Source: CAD feature listing. Evaluate the final solid. Frame: model axes, mm. Face numbers are marked on the shaded views. A direction names the side the tool comes from. Round coordinates to 2 decimals unless told otherwise and drop trailing zeros. Write each loop counter-clockwise with the first axis right and the second up, starting at its lowest first coordinate (ties: lowest second). Pieces come first, ordered by that corner, then holes. Notation, with made-up numbers: M 71.5,29 L 101.5,29 A19 ccw 101.5,45 Z; hole C -8,12.5 d10. An arc over 180 degrees is marked long. Use a Markdown table: item, result.
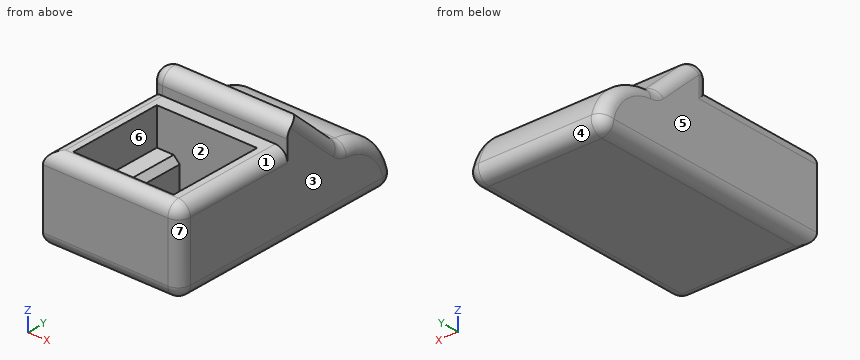
```python
from build123d import *

# Parameters (mm, degrees)
F0_W     = 57.6730370522
F0_H     = 103.7285923958
F1_DEPTH = 50.1204133034
F2_W     = 51.8642961979
F2_H     = 15.2675881982
F3_DEPTH = 280.9666395187
F4_W     = 42.251765728
F4_H     = 40.2974346653
F5_DEPTH = 28.219755739
F6_W     = 9.6290325746
F6_H     = 40.2974346653
F7_DEPTH = 12.7694699913
F8_W     = 9.6542518586
F8_H     = 40.2974346653
F9_DEPTH = 10.5208531022
F10_R    = 5.08
F11_SIZE = 2.54


with BuildPart() as f1:
    # F0 (on Top) → F1 (new body)
    with BuildSketch(Plane.XY):
        Rectangle(F0_W, F0_H)
    extrude(amount=F1_DEPTH)

    # F2 (on face) → F3 (cut)
    with BuildSketch(Plane.YZ.offset(28.8365185261)):
        with BuildLine():
            ThreePointArc((26.9694030285, 25.0602066517), (44.5827153367, 17.6618916268), (51.8642961979, 0))
            Line((51.8642961979, 0), (51.8642961979, 50.1204133034))
            Line((51.8642961979, 50.1204133034), (0, 50.1204133034))
            Line((0, 50.1204133034), (26.9694030285, 25.0602066517))
        make_face()
        with Locations((-25.9321480989, 42.4866192043)):
            Rectangle(F2_W, F2_H)
    extrude(amount=-F3_DEPTH, mode=Mode.SUBTRACT)

    # F4 (on face) → F5 (cut)
    with BuildSketch(Plane.XY.offset(34.8528251052)):
        with Locations((0, -25.9321480989)):
            Rectangle(F4_W, F4_H)
    extrude(amount=-F5_DEPTH, mode=Mode.SUBTRACT)

    # F6 (on face) → F7 (join)
    with BuildSketch(Plane.XY.offset(6.6330693662)):
        with Locations((-16.3113665767, -25.9321480989)):
            Rectangle(F6_W, F6_H)
    extrude(amount=F7_DEPTH)

    # F8 (on face) → F9 (join)
    with BuildSketch(Plane.XY.offset(6.6330693662)):
        with Locations((16.2987569347, -25.9321480989)):
            Rectangle(F8_W, F8_H)
    extrude(amount=F9_DEPTH)

    # F10
    f10_edges = [f1.edges().sort_by_distance(p)[0] for p in [
        (28.836519, 44.582715, 17.661892),
        (28.836519, 13.484702, 37.59031),
        (0, 26.969403, 25.060207),
        (-28.836519, 13.484702, 37.59031),
        (-28.836519, 44.582715, 17.661892),
        (0, 51.864296, 0),
        (28.836519, 0, 0),
        (28.836519, -25.932148, 34.852825),
        (28.836519, -51.864296, 17.426413),
        (-28.836519, -25.932148, 34.852825),
        (0, -51.864296, 34.852825),
        (0, -51.864296, 0),
        (-28.836519, 0, 0),
        (-28.836519, 0, 42.486619),
        (0, 0, 50.120413),
    ]]
    fillet(f10_edges, radius=F10_R)

    # F11
    f11_edges = [f1.edges().sort_by_distance(p)[0] for p in [
        (-11.49685, -25.932148, 19.402539),
        (11.471631, -25.932148, 17.153922),
    ]]
    chamfer(f11_edges, length=F11_SIZE)


solid = f1.part
```
Q1. Section D-D on x = -13. Return loops of the section in (y, z).
Results are:
| item | result |
|---|---|
| outline | M -51.86,5.08 A5.08 ccw -46.78,0 L 46.13,0 A5.08 ccw 51.04,6.37 A25.06 ccw 28.68,24.99 A5.08 cw 25.6,26.34 L 8.54,42.19 A5.08 ccw 0,38.47 L 0,34.85 L -5.78,34.85 L -5.78,18.37 L -46.08,18.37 L -46.08,34.85 L -46.78,34.85 A5.08 ccw -51.86,29.77 Z |
Q2. Section B-B on z = 3. Return loops of the section in (x, y), plus the area to 3 significant figures.
Results are:
| item | result |
|---|---|
| outline | M -28.39,-51.42 L 23.76,-51.42 A4.63 ccw 28.39,-46.78 L 28.39,46.13 A4.63 ccw 23.76,50.76 L -23.76,50.76 A4.63 ccw -28.39,46.13 Z |
| area | 5,790 mm^2 |
Q3. Line query: L1, parallel to X at y = -27.5, z = 20; L2, parallel to Y at x = 20, z = 27; L3, parallel to Z at x = 3.5, y = -33.5. Output: solid intervals per line, ascending.
Results are:
| item | result |
|---|---|
| L1 | -28.84 to -21.13, 21.13 to 28.84 |
| L2 | -51.86 to -46.08, -5.78 to 24.88 |
| L3 | 0 to 6.63 |
Q4. Section A-A on x = 6. Return loops of the section in (y, z), plus the area to 3 significant figures.
Results are:
| item | result |
|---|---|
| outline | M -51.86,5.08 A5.08 ccw -46.78,0 L 46.13,0 A5.08 ccw 51.04,6.37 A25.06 ccw 28.68,24.99 A5.08 cw 25.6,26.34 L 8.54,42.19 A5.08 ccw 0,38.47 L 0,34.85 L -5.78,34.85 L -5.78,6.63 L -46.08,6.63 L -46.08,34.85 L -46.78,34.85 A5.08 ccw -51.86,29.77 Z |
| area | 2,130 mm^2 |
Q5. First-contact query: pin 1 Ø5 at (y, z) = (-23.5, 36) entering from -X; pin 2 Ø6 at (y, z) = (34, 25) entering from +X; pin 3 Ø3.5 at (x, y) = (-17.5, -20.5) entering from +Z. Flat tips, straight axial feed; report the tip coordinate or a pass-through.
Results are:
| item | result |
|---|---|
| pin 1 | x = -27.21 |
| pin 2 | x = 27.83 |
| pin 3 | z = 19.4 |
Q6. Reachability of the marked faces 1, 2 and 3 from +Z, -Z, +X, -X, +Y, -Y: full face, straight path, thin tool, end or side. Return the list, or none.
Results are:
| item | result |
|---|---|
| face 1 | +Z, +X, -Y |
| face 2 | +Z |
| face 3 | +Z, -Z, +X, +Y, -Y |
Q7. Mould query, pull axis Y, two halves, no side actions, for the marked faces 4, 5, 6 and 7. Classes: +Y half, -Y half, draft (parallel to the pull), parting line (faces both ways), or undercut.
Results are:
| item | result |
|---|---|
| face 4 | +Y half |
| face 5 | draft |
| face 6 | undercut |
| face 7 | -Y half |
Q8. Section C-C on x = 22.5. Return loops of the section in (y, z), plus the area to 3 significant figures.
Results are:
| item | result |
|---|---|
| outline | M -51.86,5.08 A5.08 ccw -46.78,0 L 46.13,0 A5.08 ccw 51.04,6.37 A25.06 ccw 28.68,24.99 A5.08 cw 25.6,26.34 L 8.54,42.19 A5.08 ccw 0,38.47 L 0,34.85 L -46.78,34.85 A5.08 ccw -51.86,29.77 Z |
| area | 3,260 mm^2 |
